```python
from build123d import *

# Parameters (mm, degrees)
F1_DEPTH = 30
F2_W     = 11
F2_H     = 15
F3_DEPTH = 11
F4_W     = 15
F4_H     = 8
F5_DEPTH = 11
F6_ANGLE = -90
F8_DEPTH = 11.001


with BuildPart() as f1:
    # F0 (on Front) → F1 (new body)
    with BuildSketch(Plane.XZ):
        Polygon((0, 30), (0, 0), (40, 0), (40, 11), (11, 11), (11, 30), align=None)
    extrude(amount=F1_DEPTH)

    # F2 (on face) → F3 (cut, through all)
    with BuildSketch(Plane.XY.offset(11)):
        with Locations((34.5, -22.5)):
            Rectangle(F2_W, F2_H)
    extrude(amount=-F3_DEPTH, mode=Mode.SUBTRACT)

    # F4 (on face) → F5 (cut, through all)
    with BuildSketch(Plane.YZ.offset(11)):
        with Locations((-22.5, 26)):
            Rectangle(F4_W, F4_H)
    extrude(amount=-F5_DEPTH, mode=Mode.SUBTRACT)


with BuildPart() as f1_1:
    # F6: moved
    add(f1.part.rotate(Axis((0, 0, 15), (0, 0, 1)), F6_ANGLE))

    # F7 (on face) → F8 (cut, through all)
    with BuildSketch(Plane.XZ.offset(11)):
        Polygon((0, 30), (-15, 30), (-7.5, 26), align=None)
        Polygon((0, 30), (-7.5, 26), (0, 22), align=None)
    extrude(amount=-F8_DEPTH, mode=Mode.SUBTRACT)


solid = f1_1.part
```
Work out the finished part from the listing and answer in its coordinate system (mm). A direction names the side the tool comes from. Give positions to 0.01 mm unless a question says otherwise; leave off trailing zeros. Loops run counter-clockwise (first coordinate to the right, second up) from the corner with the lowest first, then second, coordinate; pieces in that order, holes last. Notation, with made-up numbers: (2.25, 14) - (47.25, 14) arc R12 ccw to (47.25, 35) - close; hole circle Ø1 at (-5.5, 74.25). An arc over 180 degrees is marked (long way). Use CSV: the item, a comma, the result in double quotes. Start each with the question number.
(1) Find section A-A, the plane x = -28. Determine the outline of the cut face in (y, z).
(2) A tool of negligible diameter and unlimited length cuts with its end or side. For faces 1 (the face through (-7, -40, 5)), 2 (the face through (-15, -6, 26)), 3 (the face through (-15, -11, 18)), 4 (the face through (-15, -34, 6)), from which of +Z, -Z, +X, -X, +Y, -Y can it reach the whole face along a straight path? Write none if from no direction.
(3) Find section B-B, the plane y = -6. Determine the outline of the cut face in (x, z).
(4) Each of these flat-tipped pins is pushed along its axis until it touches: pin 1 (12 mm diameter, centred on x = -24, z = 6.5, fed in from -Y); pin 2 (5.5 mm diameter, centred on y = -36, z = 7.5, fed in from -X); pin 3 (15 mm diameter, centred on x = -9, z = 25, fed in from -Y). Where does it stop, or does it pass through?
(5) Find the intervals of material crossed by L1, parallel to Z at x = -7, y = -31; L2, parallel to Y at x = -4, z = 14.5; L3, parallel to Z at x = -23, y = -5.5, in increasing order.
(6) Find section D-D, the plane y = -36.5. Determine the outline of the cut face in (x, z).
(7) Find section C-C, the plane z = 15. Determine the outline of the cut face in (x, y).
Results found:
1,outline,"(-29, 0) - (0, 0) - (0, 22) - (-11, 22) - (-11, 11) - (-29, 11) - close"
2,face 1,"+Z, -Z, +X, -X, -Y"
2,face 2,"+Z, -X, +Y, -Y"
2,face 3,"+Z, +X, -X, -Y"
2,face 4,"+Z, -Z, -X, -Y"
3,outline,"(-30, 0) - (0, 0) - (0, 22) - (-15, 30) - (-15, 22) - (-30, 22) - close"
4,pin 1,"y = -29"
4,pin 2,"x = -15"
4,pin 3,"y = -11"
5,L1,"0 to 11"
5,L2,"-11 to 0"
5,L3,"0 to 22"
6,outline,"(-15, 0) - (0, 0) - (0, 11) - (-15, 11) - close"
7,outline,"(-30, -11) - (0, -11) - (0, 0) - (-30, 0) - close"
